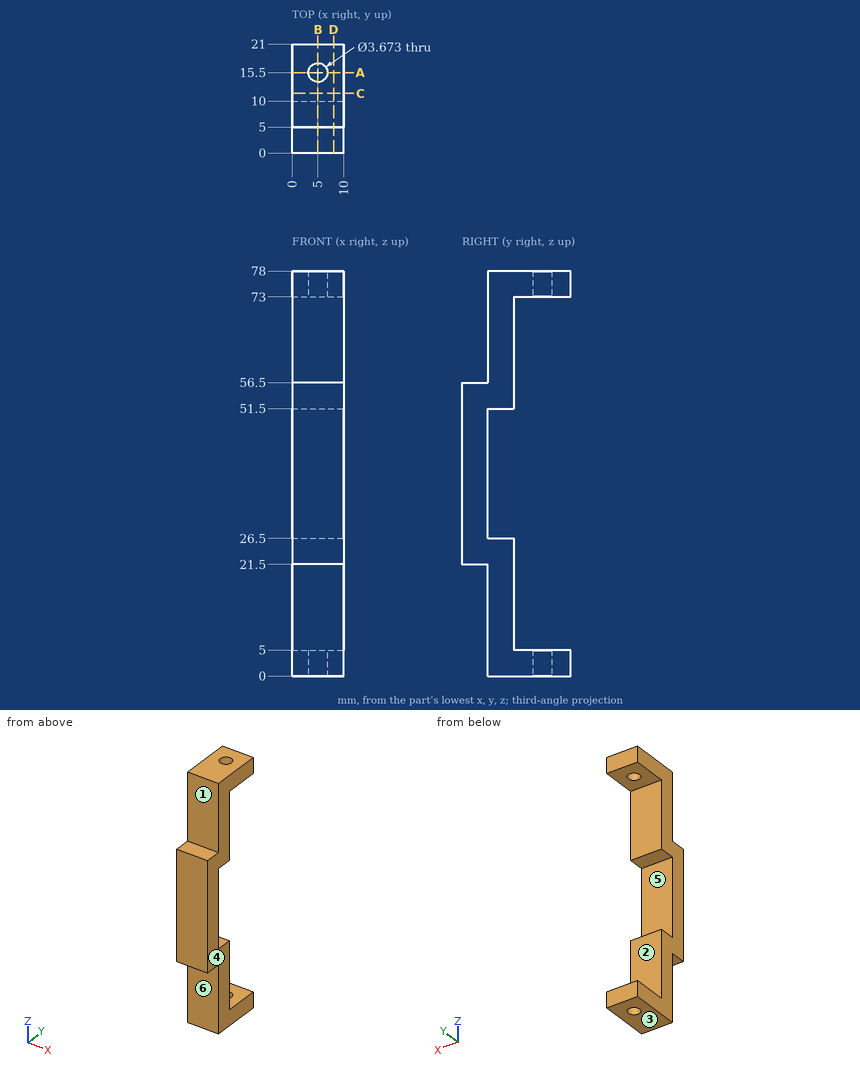
Study the drawing (mm; zero at the part's minimum x, y, z) and answer. A direction names the side the tool comes from. Give positions to 0.01 mm unless a question says otherwise; leave off trailing zeros. Loops run counter-clockwise (first coordinate to the right, second up) from the corner with the lowest first, then second, coordinate; pieces in that order, holes last. Notation, with made-up numbers: (-29, 54.25) - (26, 54.25) arc R8 cw to (26, 65.25) - close; hole circle Ø6 at (-4.5, 49). An arc over 180 degrees is marked (long way). One line per question, with ' | ' between items.
(1) The part is cut by section D-D (x = 8). Write down the section's boundary in (y, z).
Recorded:
outline: (0, 21.5) - (5, 21.5) - (5, 0) - (21, 0) - (21, 5) - (10, 5) - (10, 26.5) - (5, 26.5) - (5, 51.5) - (10, 51.5) - (10, 73) - (21, 73) - (21, 78) - (5, 78) - (5, 56.5) - (0, 56.5) - close
(2) Straight lines are drawn through the part: probe 1 along Y at (x, z) = (5, 74.95); probe 2 along Z at (x, y) = (5, 13); probe 3 along X at (y, z) = (15.5, 74.4). For each, find the intervals that lie inside material, in ascending order.
Recorded:
probe 1: y = 5 to 13.66, 17.34 to 21 | probe 2: z = 0 to 5, 73 to 78 | probe 3: x = 0 to 3.16, 6.84 to 10
(3) The part is cut by section A-A (y = 15.5). Write down the section's boundary in (x, z).
Recorded:
outline: (0, 0) - (3.16, 0) - (3.16, 5) - (0, 5) - close; (0, 73) - (3.16, 73) - (3.16, 78) - (0, 78) - close; (6.84, 0) - (10, 0) - (10, 5) - (6.84, 5) - close; (6.84, 73) - (10, 73) - (10, 78) - (6.84, 78) - close
(4) The part is cut by section C-C (y = 11.5). Write down the section's boundary in (x, z), then the cut area to 3 significant figures.
Recorded:
outline: (0, 0) - (10, 0) - (10, 5) - (0, 5) - close; (0, 73) - (10, 73) - (10, 78) - (0, 78) - close | area: 100 mm²
(5) Each of these flat-tipped pins is pushed along its axis until it touches: pin 1 Ø5 at (x, z) = (7.5, 69) entering from -Y; pin 2 Ø3 at (x, z) = (6, 58.5) entering from +Y; pin 3 Ø2.5 at (x, y) = (6.5, 1.5) entering from -Z. Where does it stop, or does it pass through?
Recorded:
pin 1: stops at y = 5 | pin 2: stops at y = 10 | pin 3: stops at z = 21.5
(6) The part is cut by section B-B (x = 5). Write down the section's boundary in (y, z).
Recorded:
outline: (0, 21.5) - (5, 21.5) - (5, 0) - (13.66, 0) - (13.66, 5) - (10, 5) - (10, 26.5) - (5, 26.5) - (5, 51.5) - (10, 51.5) - (10, 73) - (13.66, 73) - (13.66, 78) - (5, 78) - (5, 56.5) - (0, 56.5) - close; (17.34, 0) - (21, 0) - (21, 5) - (17.34, 5) - close; (17.34, 73) - (21, 73) - (21, 78) - (17.34, 78) - close
(7) The mould has two halves that part along Z. Classify the marked faces 1, 2 and 3: +Z half, -Z half, draft (parallel to the pull), parting line (faces both ways), or undercut.
Recorded:
face 1: draft | face 2: undercut | face 3: -Z half
(8) A tool of negligible diameter and unlimited length cuts with its end or side. For the marked faces 4, 5 and 6, from which of +Z, -Z, +X, -X, +Y, -Y can it reach the whole face along a straight path? Write none if from no direction.
Recorded:
face 4: +Z, -Z, +X, +Y, -Y | face 5: +X, -X, +Y | face 6: -Z, +X, -X, -Y
